Check sheet for the modelled part. Datum: model origin and axes. Units: mm. A direction names the side the tool comes from. Round coordinates to 2 decimals unless told otherwise and drop trailing zeros. Loops run counter-clockwise (first coordinate to the right, second up) from the corner with the lowest first, then second, coordinate; pieces in that order, holes last. Notation, with made-up numbers: (25, 33) - (34, 33) arc R18 ccw to (34, 63) - close; hole circle Ø2 at (78.25, 27). An arc over 180 degrees is marked (long way). Put each result on its own line as item: value.
```python
from build123d import *

# Parameters (mm, degrees)
BOSS_EXTRUDE1_DEPTH                   = 10
BOSS_EXTRUDE2_DEPTH                   = 22
F_12_0MM_DOWEL_HOLE1_D                = 12
F_12_0MM_DOWEL_HOLE1_DEPTH            = 20.394836286
F_12_0MM_DOWEL_HOLE1_TIP              = 3.605163714
TAP_DRILL_FOR_M6X1_0_TAP1_D           = 5
TAP_DRILL_FOR_M6X1_0_TAP1_DEPTH       = 16
TAP_DRILL_FOR_M6X1_0_TAP1_TIP         = 1.502151548
TAP_DRILL_FOR_M6X1_0_TAP3_D           = 5
TAP_DRILL_FOR_M6X1_0_TAP3_DEPTH       = 16
TAP_DRILL_FOR_M6X1_0_TAP3_CSINK_D     = 5.05
TAP_DRILL_FOR_M6X1_0_TAP3_CSINK_ANGLE = 100
TAP_DRILL_FOR_M6X1_0_TAP3_TIP         = 1.502151548
SKETCH13_R                            = 6
CUT_EXTRUDE1_DEPTH                    = 4


with BuildPart() as part:
    # Sketch1 → Boss-Extrude1 (new body)
    with BuildSketch(Plane.XY):
        Polygon((-32, 9), (-8, 9), (-8, 0), (8, 0), (8, 9), (32, 9), (32, 45), (-32, 45), align=None)
    extrude(amount=BOSS_EXTRUDE1_DEPTH)

    # Sketch3 → Boss-Extrude2 (add)
    with BuildSketch(Plane.XY.offset(10)):
        with BuildLine():
            Line((-32, 19), (-32, 9))
            Line((-32, 9), (-8, 9))
            Line((-8, 9), (-8, 0))
            Line((-8, 0), (8, 0))
            Line((8, 0), (8, 9))
            Line((8, 9), (32, 9))
            Line((32, 9), (32, 19))
            Line((32, 19), (22.317123285, 19))
            Line((22.317123285, 19), (14.500924593, 35.761892188))
            ThreePointArc((14.500924593, 35.761892188), (8.596793696, 42.494263157), (-8.8e-08, 45))
            ThreePointArc((-8.8e-08, 45), (-8.596793771, 42.494263109), (-14.500924593, 35.761892188))
            Line((-14.500924593, 35.761892188), (-22.317123285, 19))
            Line((-22.317123285, 19), (-32, 19))
        make_face()
    extrude(amount=BOSS_EXTRUDE2_DEPTH)

    # Ø12.0mm Dowel Hole1
    with Locations(Plane.XY.offset(32)):
        with Locations((0, 29)):
            Hole(F_12_0MM_DOWEL_HOLE1_D / 2, depth=F_12_0MM_DOWEL_HOLE1_DEPTH)
            with Locations((0, 0, -(F_12_0MM_DOWEL_HOLE1_DEPTH + F_12_0MM_DOWEL_HOLE1_TIP / 2))):  # 118° drill point
                Cone(0, F_12_0MM_DOWEL_HOLE1_D / 2, F_12_0MM_DOWEL_HOLE1_TIP, mode=Mode.SUBTRACT)

    # Tap Drill for M6x1.0 Tap1
    with Locations(Plane(origin=(0, 0, 0), x_dir=(-1, 0, 0), z_dir=(0, -1, 0))):
        with Locations((0, -8), (0, -24)):
            Hole(TAP_DRILL_FOR_M6X1_0_TAP1_D / 2, depth=TAP_DRILL_FOR_M6X1_0_TAP1_DEPTH)
            with Locations((0, 0, -(TAP_DRILL_FOR_M6X1_0_TAP1_DEPTH + TAP_DRILL_FOR_M6X1_0_TAP1_TIP / 2))):  # 118° drill point
                Cone(0, TAP_DRILL_FOR_M6X1_0_TAP1_D / 2, TAP_DRILL_FOR_M6X1_0_TAP1_TIP, mode=Mode.SUBTRACT)

    # Tap Drill for M6x1.0 Tap3
    with Locations(Plane(origin=(0, 45, 20), x_dir=(1, 0, 0), z_dir=(0, 1, 0))):
        with Locations((0, 0)):
            CounterSinkHole(TAP_DRILL_FOR_M6X1_0_TAP3_D / 2, TAP_DRILL_FOR_M6X1_0_TAP3_CSINK_D / 2, depth=TAP_DRILL_FOR_M6X1_0_TAP3_DEPTH, counter_sink_angle=TAP_DRILL_FOR_M6X1_0_TAP3_CSINK_ANGLE)
            with Locations((0, 0, -(TAP_DRILL_FOR_M6X1_0_TAP3_DEPTH + TAP_DRILL_FOR_M6X1_0_TAP3_TIP / 2))):  # 118° drill point
                Cone(0, TAP_DRILL_FOR_M6X1_0_TAP3_D / 2, TAP_DRILL_FOR_M6X1_0_TAP3_TIP, mode=Mode.SUBTRACT)

    # Sketch13 → Cut-Extrude1 (cut)
    with BuildSketch(Plane(origin=(0, 45, 0), x_dir=(1, 0, 0), z_dir=(0, 1, 0))):
        with Locations((0, -20)):
            Circle(SKETCH13_R)
    extrude(amount=-CUT_EXTRUDE1_DEPTH, mode=Mode.SUBTRACT)


solid = part.part
```
Item 1: Thickness scan on line 1 (Z direction, x = 0, y = 4.5); line 2 (Z direction, x = 0, y = 43.55); line 3 (Y direction, x = 0, z = 27). Record the ranges inside material, lowest first. Write a range as from..to.
Filled sheet:
line 1: 0..5.5, 10.5..21.5, 26.5..32
line 2: 0..14, 26..32
line 3: 0..23, 35..45
Item 2: Section check C-C on x = -7. Enter the section's corners in (y, z).
Filled sheet:
outline: (0, 0) - (45, 0) - (45, 10) - (43.39, 10) - (43.39, 32) - (0, 32) - close
Item 3: Tool access check on faces 1 (the cylindrical face through (2.5, 37.7, 19.9)), 2 (the flat face through (-18.354, 27.498, 20.846)), 3 (the flat face through (-20, 9, 16)), 4 (the flat face through (20, 9, 16)). Record the directions out of +Z, -Z, +X, -X, +Y, -Y that give a thin tool (end or side, any length) a straight path to the whole face; none if there is none.
Filled sheet:
face 1: +Y
face 2: +Z, -X, +Y
face 3: +Z, -Z, -X, -Y
face 4: +Z, -Z, +X, -Y
Item 4: Section check B-B on x = 26. Enter the section's corners in (y, z).
Filled sheet:
outline: (9, 0) - (45, 0) - (45, 10) - (19, 10) - (19, 32) - (9, 32) - close
Item 5: Release check for a two-part mould opening along X. For faces 5 (the flat face through (-8, 5, 16)), 6 (the flat face through (0, 45, 5)), 7 (the flat face through (0, 41, 23)), 8 (the flat face through (18.464, 27.264, 20.846)) record: +X half, -X half, draft (parallel to the pull), parting line (faces both ways), or undercut.
Filled sheet:
face 5: -X half
face 6: draft
face 7: undercut
face 8: +X half
Item 6: Go/stop test with flat-tipped pins: pin 1 (4.5 mm diameter, centred on x = 0, z = 8, fed in from -Y); pin 2 (10.5 mm diameter, centred on x = -27.5, z = 22, fed in from +Y); pin 3 (5 mm diameter, centred on x = 1, z = 23.5, fed in from +Y). Record where each tip stops, or that it passes through.
Filled sheet:
pin 1: y = 16.15
pin 2: y = 19.14
pin 3: y = 44.99
Item 7: Section check A-A on z = 20. Enter the section's corners in (x, y), then the cut area to 3 significant figures.
Filled sheet:
outline: (-32, 9) - (-8, 9) - (-8, 0) - (8, 0) - (8, 9) - (32, 9) - (32, 19) - (22.32, 19) - (14.5, 35.76) arc R16 ccw to (6, 43.83) - (6, 41) - (2.5, 41) - (2.5, 34.45) arc R6 cw (long way) to (-2.5, 34.45) - (-2.5, 41) - (-6, 41) - (-6, 43.83) arc R16 ccw to (-14.5, 35.76) - (-22.32, 19) - (-32, 19) - close
area: 1,410 mm²
